The listing builds one solid part. Answer for the finished solid, in the listing's coordinates (mm). A direction names the side the tool comes from. Give positions to 0.01 mm unless a question says otherwise; leave off trailing zeros. Order: outer loops, then holes, each group sorted by start corner. A loop starts at its lowest first (then second) coordinate and runs counter-clockwise, first axis right, second up. Notation, with made-up numbers: (-21, 20) - (10, 20) arc R29 ccw to (10, 47) - close; hole circle Ø9 at (62.25, -12). An arc over 180 degrees is marked (long way). Answer as a JSON object with one key per item and string values. Group by question number.
Q1. A cutting plane is placed at A-A, the plane z = 2. Give the vertices of the cut face in (x, y).
Q2. A cutting plane is placed at B-B, the plane y = 54. Give the vertices of the cut face in (x, z), and give its area (3 significant figures).
Q3. Consider line 1 (Y direction, x = 14, z = 2.35); line 2 (X direction, y = -38.5, z = 2.35); line 3 (Z direction, x = 23.7, y = 0). Determine where each line is inside the solid, lowest interval first.
Q4. The mould has two halves that part along X. Classify faces 3 (the face through (0, -75, 2)), 4 (the face through (0, 73, 2)), 5 (the face through (25, -1.05, 1.53)): released by +X, released by -X, zero draft, split by the parting line, or undercut.
Q5. Given pin 1 (1.8 mm diameter, centred on y = 49.5, z = 2, fed in from +X); pin 2 (10 mm diameter, centred on x = 16.5, y = -13, fed in from -Z), each flat-ended and moving along its own axis, determine where each tip first touches the part or whether it passes through.
Q6. A cutting plane is placed at C-C, the plane x = -17. Give the vertices of the cut face in (y, z).
Q7. For faces 1 (the face through (-23, 24, 2)), 2 (the face through (24, 0, 0)), determine the directions among +Z, -Z, +X, -X, +Y, -Y from which every point of the face is accessible in a straight line to the end or side of a thin tool.
from build123d import *

# Parameters (mm, degrees)
F0_W     = 50
F0_H     = 150
F0_W_2   = 46
F0_H_2   = 47
F0_H_3   = 97
F1_DEPTH = 4
F2_R     = 1
F3_DEPTH = 25


with BuildPart() as f1:
    # F0 (on Top) → F1 (new body)
    with BuildSketch(Plane.XY):
        Rectangle(F0_W, F0_H)
        with Locations((0, -49.5)):
            Rectangle(F0_W_2, F0_H_2, mode=Mode.SUBTRACT)
        with Locations((0, 24.5)):
            Rectangle(F0_W_2, F0_H_3, mode=Mode.SUBTRACT)
    extrude(amount=F1_DEPTH)

    # F2 (on face) → F3 (cut)
    with BuildSketch(Plane.YZ.offset(25)):
        with Locations((-49.5, 2)):
            Circle(F2_R)
        with Locations((0, 2)):
            Circle(F2_R)
        with Locations((49.5, 2)):
            Circle(F2_R)
    extrude(amount=-F3_DEPTH, mode=Mode.SUBTRACT)


solid = f1.part
Reply:
{
 "1": {"outline": "(-25, -75) - (25, -75) - (25, -50.5) - (23, -50.5) - (23, -73) - (-23, -73) - (-23, -26) - (23, -26) - (23, -48.5) - (25, -48.5) - (25, -1) - (23, -1) - (23, -24) - (-23, -24) - (-23, 73) - (23, 73) - (23, 50.5) - (25, 50.5) - (25, 75) - (-25, 75) - close; (23, 1) - (25, 1) - (25, 48.5) - (23, 48.5) - close"},
 "2": {"outline": "(-25, 0) - (-23, 0) - (-23, 4) - (-25, 4) - close; (23, 0) - (25, 0) - (25, 4) - (23, 4) - close", "area": "16.0 mm^2"},
 "3": {"line 1": "y = -75 to -73, -26 to -24, 73 to 75", "line 2": "x = -25 to -23, 23 to 25", "line 3": "z = 0 to 1, 3 to 4"},
 "4": {"face 3": "zero draft", "face 4": "undercut", "face 5": "released by +X"},
 "5": {"pin 1": "stops at x = -23", "pin 2": "passes through"},
 "6": {"outline": "(-75, 0) - (-73, 0) - (-73, 4) - (-75, 4) - close; (-26, 0) - (-24, 0) - (-24, 4) - (-26, 4) - close; (73, 0) - (75, 0) - (75, 4) - (73, 4) - close"},
 "7": {"face 1": "+Z, -Z", "face 2": "-Z, +X, -X, +Y, -Y"}
}
